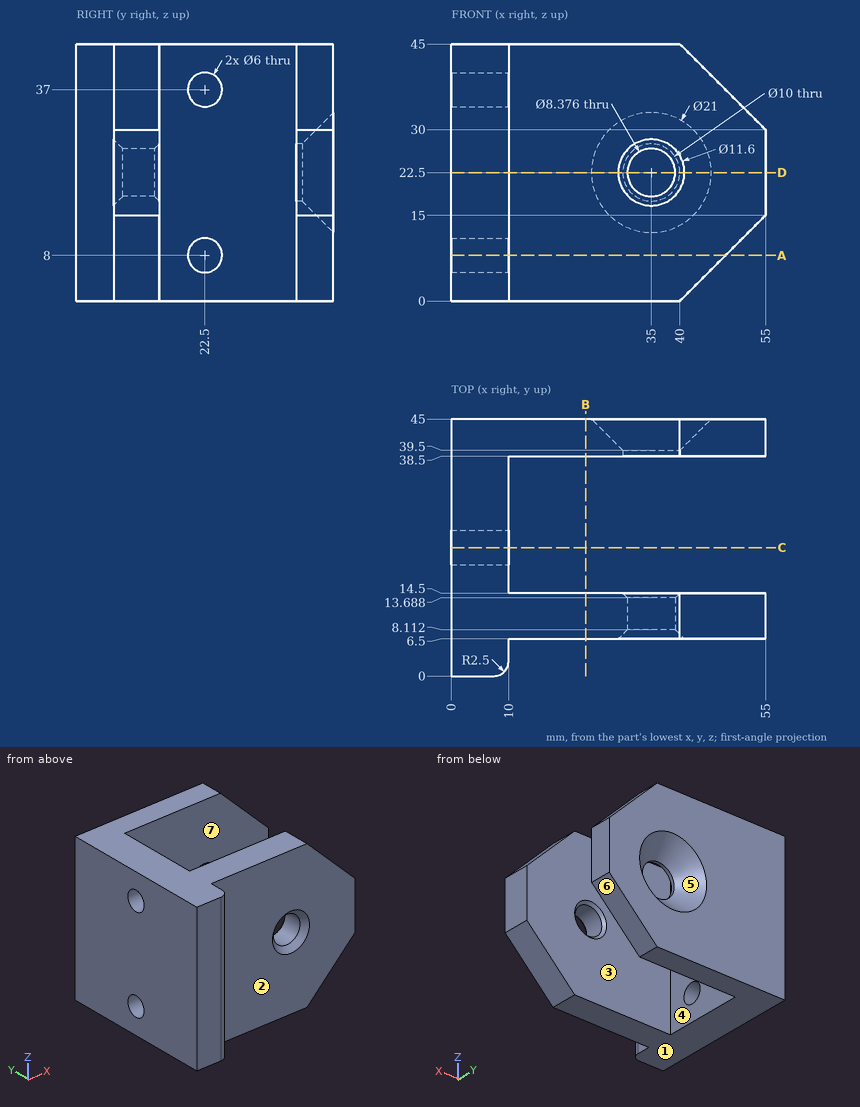
For this review, use the dimensioned drawing (mm, ordinates from the lowest corner) and the shaded views. A direction names the side the tool comes from. Give positions to 0.01 mm unless a question says otherwise; leave off trailing zeros. Order: outer loops, then holes, each group sorted by start corner. A loop starts at its lowest first (then second) coordinate and runs counter-clockwise, first axis right, second up.
1) Insertion check: pin 1 (10 mm diameter, centred on y = 27, z = 25.5, fed in from +X); pin 2 (22.5 mm diameter, centred on x = 32.5, z = 16, fed in from -Y). Each pin has a flat end and moves straight along its axis. Give the tip position at first contact, or say it passes through.
2) Take a section at B-B (x = 23.5). Give the boundary of the cut face in (y, z), then the cut area to 4 significant figures.
3) The part is to be moulded in two halves that separate along Y. For the marked faces 4, 5, 6 and 7, say which applies: released by +Y, released by -Y, zero draft, split by the parting line, or undercut.
4) Take a section at A-A (z = 8). Give the boundary of the cut face in (x, y), then the cut area to 3 significant figures.
5) Take a section at D-D (z = 22.5). Give the boundary of the cut face in (x, y).
6) For the marked faces 1, 2 and 3, list the 3-axis set-ups (+Z, -Z, +X, -X, +Y, -Y) from which the entire face can be reached by the end or side of a thin tool; tool diameter is ignored.
7) Wall thickness on line 1 (Y direction, x = 4, z = 37); line 2 (X direction, y = 39.2, z = 22.5); line 3 (X direction, y = 32, z = 4): over which ranges is each line inside the solid? List them lowest first.
8) Take a section at C-C (y = 22.5). Give the boundary of the cut face in (x, z).
Derived:
1. pin 1: stops at x = 10
1. pin 2: stops at y = 6.5
2. outline: (6.5, 0) - (14.5, 0) - (14.5, 45) - (6.5, 45) - close; (38.5, 0) - (45, 0) - (45, 45) - (38.5, 45) - close
2. area: 652.5 mm2
3. face 4: undercut
3. face 5: released by +Y
3. face 6: zero draft
3. face 7: undercut
4. outline: (0, 0) - (7.5, 0) arc R2.5 ccw to (10, 2.5) - (10, 6.5) - (48, 6.5) - (48, 14.5) - (10, 14.5) - (10, 19.5) - (0, 19.5) - close; (0, 25.5) - (10, 25.5) - (10, 38.5) - (48, 38.5) - (48, 45) - (0, 45) - close
4. area: 940 mm2
5. outline: (0, 0) - (7.5, 0) arc R2.5 ccw to (10, 2.5) - (10, 6.5) - (29.2, 6.5) - (30.81, 8.11) - (30.81, 13.69) - (30, 14.5) - (10, 14.5) - (10, 38.5) - (30, 38.5) - (30, 39.5) - (24.5, 45) - (0, 45) - close; (39.19, 8.11) - (40.8, 6.5) - (55, 6.5) - (55, 14.5) - (40, 14.5) - (39.19, 13.69) - close; (40, 38.5) - (55, 38.5) - (55, 45) - (45.5, 45) - (40, 39.5) - close
6. face 1: -Z, +X, -X, +Y, -Y
6. face 2: +Z, -Z, +X, -Y
6. face 3: +Z, -Z, +X
7. line 1: y = 0 to 19.5, 25.5 to 45
7. line 2: x = 0 to 30, 40 to 55
7. line 3: x = 0 to 10
8. outline: (0, 0) - (10, 0) - (10, 5) - (0, 5) - close; (0, 11) - (10, 11) - (10, 34) - (0, 34) - close; (0, 40) - (10, 40) - (10, 45) - (0, 45) - close
